The listing builds one solid part. Answer for the finished solid, in the listing's coordinates (mm). A direction names the side the tool comes from. Round coordinates to 2 decimals unless told otherwise and drop trailing zeros. Write each loop counter-clockwise with the first axis right and the second up, starting at its lowest first coordinate (ties: lowest second). Pieces come first, ordered by that corner, then holes.
(1) Find the intervals of material crossed by probe 1 along Y at (x, z) = (47, 13); probe 2 along Z at (x, y) = (52, 6); probe 3 along X at (y, z) = (31, 9.75), in increasing order.
(2) Each of these flat-tipped pins is pushed along its axis until it touches: pin 1 Ø1.5 at (x, y) = (36, 11.5) entering from -Z; pin 2 Ø4 at (y, z) = (34, 11) entering from -X; pin 3 Ø6.5 at (x, z) = (44.5, 7.5) entering from +Y; pin 4 Ø6.5 at (y, z) = (8, 8.5) entering from +X. Where does it stop, or does it pass through?
(3) A cutting plane is placed at D-D, the plane y = 43. Give the vertices of the cut face in (x, z).
(4) For faces 4 (the face through (48, 0.731, 7)), 5 (the face through (38.32, 32.62, 8.1)), 6 (the face through (51.3, 32, 7.4)), determine the directions among +Z, -Z, +X, -X, +Y, -Y from which every point of the face is accessible in a straight line to the end or side of a thin tool.
(5) A cutting plane is placed at A-A, the plane z = 2.5. Give the vertices of the cut face in (x, y).
(6) The mould has two halves that part along Y. Classify faces 1 (the face through (39, 15, 15)), 2 (the face through (47.366, 42.127, 7.395)), 3 (the face through (18.65, 1.06, 7.4)): +Y half, -Y half, draft (parallel to the pull), parting line (faces both ways), or undercut.
(7) A cutting plane is placed at B-B, the plane x = 25. Give the vertices of the cut face in (y, z), and give its area (3 significant figures).
(8) A cutting plane is placed at C-C, the plane y = 27.5. Give the vertices of the cut face in (x, z), and give its area (3 significant figures).
Autodesk Inventor part; units mm, degrees
ref_plane "YZ Plane" through (0, 0, 0) normal (1, 0, 0) x (0, 1, 0)
ref_plane "XZ Plane" through (0, 0, 0) normal (0, 1, 0) x (-1, 0, 0)
ref_plane "XY Plane" through (0, 0, 0) normal (0, 0, 1) x (1, 0, 0)
sketch "Sketch1" plane through (0, 0, 0) normal (0, 0, 1) x (1, 0, 0)
  line L0 (26, 0) -> (52, 0)
  circle A0 centre (46.5768, 46.5768) radius 2.4
  arc A1 (48.4457, 43.7365) -> (43.7365, 48.4457) centre (46.5768, 46.5768) ccw
  arc A2 (3.5543, 8.2635) -> (8.2635, 3.5543) centre (5.4232, 5.4232) ccw
  circle A3 centre (5.4232, 5.4232) radius 2.4
  line L1 (55, 0) -> (55, 20)
  arc A4 (40.2754, 47.7304) -> (43.7365, 48.4457) centre (41.6481, 49.8199) ccw
  arc A5 (48.4457, 43.7365) -> (47.7304, 40.2754) centre (49.8199, 41.6481) ccw
  arc A6 (40.2754, 47.7304) -> (4.2696, 11.7246) centre (26, 26) ccw
  arc A7 (11.7246, 4.2696) -> (8.2635, 3.5543) centre (10.3519, 2.1801) ccw
  arc A8 (3.5543, 8.2635) -> (4.2696, 11.7246) centre (2.1801, 10.3519) ccw
  arc A9 (11.7246, 4.2696) -> (26, 0) centre (26, 26) ccw
  arc A10 (51.8032, 22.807) -> (47.7304, 40.2754) centre (26, 26) ccw
  arc A11 (51.8032, 22.807) -> (54.2843, 20) centre (54.2843, 22.5) ccw
  line L2 (55, 0) -> (52, 0)
  line L3 (55, 20) -> (54.2843, 20)
  point P0 (48.981, 48.981)
  dimension "d6" = 4.8
  dimension "d7" = 29
  dimension "d8" = 20
  dimension "d9" = 2.5
  dimension "d10" = 2.5
  dimension "d11" = 2.5
extrude "Extrusion1" add sketch "Sketch1" along normal blind 15
sketch "Sketch2" plane through (55, 0, 0) normal (1, 0, 0) x (0, 0, -1)
  line L0 (-14.1994, 18.9903) -> (-0.92, 18.9903)
  line L1 (-0.92, 18.9903) -> (-0.92, 0.7311)
  line L2 (-0.92, 0.7311) -> (-14.1994, 0.7311)
  line L3 (-14.1994, 0.7311) -> (-14.1994, 18.9903)
extrude "Extrusion2" cut sketch "Sketch2" against normal blind 15
sketch "Sketch3" plane through (0, 0, 15) normal (0, 0, 1) x (1, 0, 0)
  circle A0 centre (26.8751, 29.0108) radius 12
  circle A1 centre (26.8751, 29.0108) radius 16
  point P0 (0, 0)
  dimension "d16" = 24
  dimension "d18" = 32
extrude "Extrusion3" cut sketch "Sketch3" against normal blind 14
properties part number "blowerFan50x15"
Solutions:
1. probe 1: y = 0 to 0.73, 18.99 to 44.21, 48.94 to 49.95
1. probe 2: z = 0 to 0.92, 14.2 to 15
1. probe 3: x = 0.49 to 11, 15.04 to 38.71, 42.75 to 51.51
2. pin 1: stops at z = 0
2. pin 2: stops at x = 0.7
2. pin 3: stops at y = 49.98
2. pin 4: stops at x = 40
3. outline: (6.33, 0) - (47.72, 0) - (47.72, 15) - (34.64, 15) - (34.64, 1) - (19.11, 1) - (19.11, 15) - (6.33, 15) - close
4. face 4: +X
4. face 5: +Z
4. face 6: +Z, -Z, +X
5. outline: (3.55, 8.26) arc R3.4 ccw (long way) to (8.26, 3.55) arc R2.5 cw to (11.72, 4.27) arc R26 ccw to (26, 0) - (55, 0) - (55, 0.73) - (40, 0.73) - (40, 18.99) - (55, 18.99) - (55, 20) - (54.28, 20) arc R2.5 cw to (51.8, 22.81) arc R26 ccw to (47.73, 40.28) arc R2.5 cw to (48.45, 43.74) arc R3.4 ccw (long way) to (43.74, 48.45) arc R2.5 cw to (40.28, 47.73) arc R26 ccw to (4.27, 11.72) arc R2.5 cw to start; circle Ø24 at (26.88, 29.01); hole circle Ø4.8 at (5.42, 5.42); hole circle Ø32 at (26.88, 29.01); hole circle Ø4.8 at (46.58, 46.58)
6. face 1: draft
6. face 2: undercut
6. face 3: -Y half
7. outline: (0.02, 0) - (51.98, 0) - (51.98, 15) - (44.9, 15) - (44.9, 1) - (40.86, 1) - (40.86, 15) - (17.16, 15) - (17.16, 1) - (13.12, 1) - (13.12, 15) - (0.02, 15) - close
7. area: 666 mm2
8. outline: (0.04, 0) - (51.96, 0) - (51.96, 15) - (42.8, 15) - (42.8, 1) - (38.78, 1) - (38.78, 15) - (14.97, 15) - (14.97, 1) - (10.95, 1) - (10.95, 15) - (0.04, 15) - close
8. area: 666 mm2
